Read the model definition and answer for the solid it produces. Units are mm, in the model's axes. A direction names the side the tool comes from. Give positions to 0.01 mm unless a question says otherwise; leave off trailing zeros. Order: outer loops, then holes, each group sorted by start corner. A loop starts at its lowest first (then second) coordinate and runs counter-clockwise, first axis right, second up. Notation, with made-up numbers: (61.5, 56.25) - (116.5, 56.25) arc R19 cw to (116.5, 69.25) - close; hole circle Ø1 at (47, 4). An arc over 180 degrees is marked (long way). Use a Markdown table: item, result. Add a question column.
1. A cutting plane is placed at B-B on z = 1.75. Determine the outline of the cut face in (x, y).
2. Consider L1, parallel to X at y = 6.5, z = -0.5; L2, parallel to Y at x = -19.5, z = -2.5; L3, parallel to Y at x = -16.75, z = -1.5. Determine where each line is inside the solid, lowest interval first.
3. Which of the six approach directions +Z, -Z, +X, -X, +Y, -Y give full straight-line access (tool end or side, diameter ignored) to faces 4 (the flat face through (-24.924, -20, 0)), 5 (the cylindrical face through (-16.416, 14.127, 0.751)), 6 (the flat face through (-24.1, -13.66, 0.05)), 7 (the flat face through (-14, 6, 3.6)), 8 (the flat face through (-20, -19.139, 0))?
4. A cutting plane is placed at D-D on y = -15.5. Determine the outline of the cut face in (x, z).
5. For a pull along Z with two mould halves and no side action, classify faces 1 (the flat face through (-12.595, 1, 0)), 2 (the flat face through (-14, 6, -3.6)), 3 (the flat face through (-19, 15.064, 0)) as released by +Z, released by -Z, zero draft, split by the parting line, or undercut.
6. A flat-ended cylindrical pin translates along its axis: P1, Ø1, axis at x = -15, z = -1, coming from the +Y side. Find the tip coordinate at first contact, or state that the pin passes through.
7. A cutting plane is placed at C-C on x = -24. Determine the outline of the cut face in (y, z), and give its area (3 significant figures).
8. A cutting plane is placed at A-A on y = 9. Determine the outline of the cut face in (x, z).
```python
from build123d import *

# Parameters (mm, degrees)
F0_R     = 2.5
F1_DEPTH = 3.6
F2_W     = 9
F2_H     = 7.2
F2_R     = 2.5
F3_DEPTH = 0.8
F4_DEPTH = 1.9


with BuildPart() as f1:
    # F0 (on Top) → F1 (new body, symmetric)
    with BuildSketch(Plane.XY):
        Polygon((-23.254177, -13.525072), (-23.254177, 15.064048), (-14.254177, 15.064048), (-14.254177, -19.138907), (-24.92434, -19.138907), (-24.92434, -20.359321), (-12.594674, -20.359321), (-12.594674, 21.997963), (-24.92434, 22.119868), (-24.92434, -13.792475), align=None)
        with Locations((-18.754847, 18.500099)):
            Circle(F0_R, mode=Mode.SUBTRACT)
    extrude(amount=F1_DEPTH, both=True)

    # F2 (on face) → F3 (join)
    with BuildSketch(Plane.XZ.offset(-15.064048)):
        with Locations((-18.754177, 0)):
            Rectangle(F2_W, F2_H)
        with Locations((-18.800411, 0)):
            Circle(F2_R, mode=Mode.SUBTRACT)
    extrude(amount=F3_DEPTH)

    # F2 (on face) → F4 (join)
    with BuildSketch(Plane.XZ.offset(-15.064048)):
        with Locations((-18.754177, 0)):
            Rectangle(F2_W, F2_H)
        with Locations((-18.800411, 0)):
            Circle(F2_R, mode=Mode.SUBTRACT)
    extrude(amount=F4_DEPTH)


solid = f1.part
```
Output values:
| question | item | result |
|---|---|---|
| 1 | outline | (-24.92, -20.36) - (-12.59, -20.36) - (-12.59, 22) - (-24.92, 22.12) - (-24.92, -13.79) - (-23.25, -13.53) - (-23.25, 13.16) - (-20.59, 13.16) - (-20.59, 15.06) - (-17.02, 15.06) - (-17.02, 13.16) - (-14.25, 13.16) - (-14.25, -19.14) - (-24.92, -19.14) - close; hole circle Ø5 at (-18.75, 18.5) |
| 2 | L1 | -24.92 to -23.25, -14.25 to -12.59 |
| 2 | L2 | -20.36 to -19.14, 13.16 to 16.11, 20.89 to 22.07 |
| 2 | L3 | -20.36 to -19.14, 13.16 to 17.01, 19.99 to 22.04 |
| 3 | face 4 | +Z, -Z, -X, +Y, -Y |
| 3 | face 5 | none |
| 3 | face 6 | +Z, -Z |
| 3 | face 7 | +Z, +X, -X, +Y, -Y |
| 3 | face 8 | +Z, -Z, -X |
| 4 | outline | (-14.25, -3.6) - (-12.59, -3.6) - (-12.59, 3.6) - (-14.25, 3.6) - close |
| 5 | face 1 | zero draft |
| 5 | face 2 | released by -Z |
| 5 | face 3 | undercut |
| 6 | P1 | y = 22.03 |
| 7 | outline | (-20.36, -3.6) - (-19.14, -3.6) - (-19.14, 3.6) - (-20.36, 3.6) - close; (-13.64, -3.6) - (22.11, -3.6) - (22.11, 3.6) - (-13.64, 3.6) - close |
| 7 | area | 266 mm² |
| 8 | outline | (-24.92, -3.6) - (-23.25, -3.6) - (-23.25, 3.6) - (-24.92, 3.6) - close; (-14.25, -3.6) - (-12.59, -3.6) - (-12.59, 3.6) - (-14.25, 3.6) - close |
